```python
from build123d import *

# Parameters (mm, degrees)
BOX_W                  = 313
BOX_H                  = 200
BOX_DEPTH              = 37
BOX_PLACEMENT_ANGLE    = 45
BOX008_W               = 200
BOX008_H               = 200
BOX008_DEPTH           = 33
CUT007_PLACEMENT_ANGLE = 45


with BuildPart() as cube002:
    # Box → Box (new body)
    with BuildSketch(Plane.XY):
        with Locations((156.5, 100)):
            Rectangle(BOX_W, BOX_H)
    extrude(amount=BOX_DEPTH)


with BuildPart() as cube002_1:
    # Box placement: moved
    add(cube002.part.moved(Location((0, 0, -2))).rotate(Axis((0, 0, -2), (0, 0, 1)), BOX_PLACEMENT_ANGLE))


with BuildPart() as short_45a:
    # Box008 → Box008 (new body)
    with BuildSketch(Plane.XY.offset(-1)):
        with Locations((100, 100)):
            Rectangle(BOX008_W, BOX008_H)
    extrude(amount=BOX008_DEPTH)

    # Cut007: cut Cube002
    add(cube002_1.part, mode=Mode.SUBTRACT)


with BuildPart() as short_45a_1:
    # Cut007 placement: moved
    add(short_45a.part.rotate(Axis((0, 0, 0), (0, 0, 1)), CUT007_PLACEMENT_ANGLE))


solid = short_45a_1.part
```
CAD build for the part. Positions are in the model's coordinates, mm. Coordinates: 2 decimals unless noted, no trailing zeros. Order: outer loops, then holes, each group sorted by start corner. A loop starts at its lowest first (then second) coordinate and runs counter-clockwise, first axis right, second up. Notation, with made-up numbers: (86, -19) - (92, -19) arc R13 ccw to (92, -1) - close; hole circle Ø4 at (-12.75, -16). An arc over 180 degrees is marked (long way). Answer in a Markdown table with one row per item.
1. Slice it at A-A, the plane z = 20. List the corners of the cut face in (x, y).
Answer:
| item | result |
|---|---|
| outline | (0, 0) - (141.42, 141.42) - (0, 282.84) - close |
2. Slice it at C-C, the plane x = 96.5. List the corners of the cut face in (y, z), then the cut area to 3 significant figures.
Answer:
| item | result |
|---|---|
| outline | (96.5, -1) - (186.34, -1) - (186.34, 32) - (96.5, 32) - close |
| area | 2,960 mm² |
3. Pull direction X, two halves, no side cores. Call faces 1 (the face through (71.7, 211.14, 15.27)), 2 (the face through (61, 141, 32)), 3 (the face through (0, 139, 15)): +X half, -X half, draft (parallel to the pull), parting line (faces both ways), or undercut.
Answer:
| item | result |
|---|---|
| face 1 | +X half |
| face 2 | draft |
| face 3 | -X half |
4. Slice it at B-B, the plane y = 50. List the corners of the cut face in (x, z), then the cut area to 3 significant figures.
Answer:
| item | result |
|---|---|
| outline | (0, -1) - (50, -1) - (50, 32) - (0, 32) - close |
| area | 1,650 mm² |
5. Flat gauge pins, fed straight in: P1, Ø12, axis at x = 51, z = 20.5, coming from the -Y side; P2, Ø1, axis at y = 41.5, z = 21, coming from the +X side; P3, Ø6, axis at x = 35, z = 24, coming from the -Y side. Where does each tip first touch, or does it go through?
Answer:
| item | result |
|---|---|
| P1 | y = 45 |
| P2 | x = 42 |
| P3 | y = 32 |
6. Drill centre lines: L1, parallel to Y at x = 26.5, z = 14; L2, parallel to X at y = 146.5, z = 27; L3, parallel to Y at x = 90, z = 13. Where is each one in solid material? Low to high. Write a range as from..to.
Answer:
| item | result |
|---|---|
| L1 | 26.5..256.34 |
| L2 | 0..136.34 |
| L3 | 90..192.84 |
